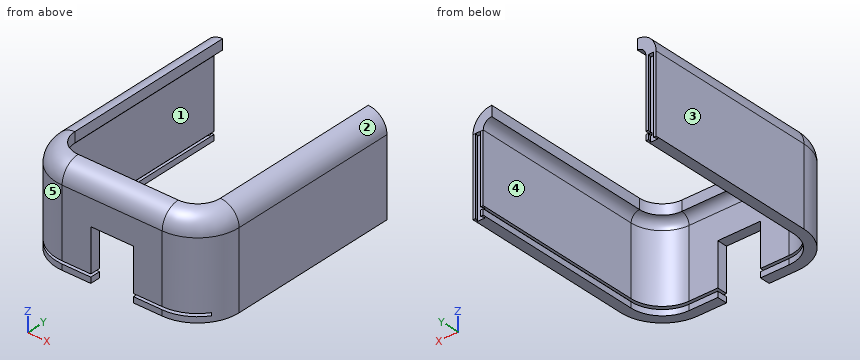
from build123d import *

# Parameters (mm, degrees)
EXTRUDE_1_DEPTH     = 27
CUT_EXTRUDE_1_DEPTH = 1
SKETCH_4_W          = 15
SKETCH_4_H          = 3.6
CUT_EXTRUDE_2_DEPTH = 6
SKETCH_4_2_W        = 15
SKETCH_4_2_H        = 3.6
CUT_EXTRUDE_3_DEPTH = 13


with BuildPart() as part:
    # Sketch 1 → Extrude 1 (new body)
    with BuildSketch(Plane.XY):
        with BuildLine():
            Line((-17.6, -33.659429503), (17.6, -33.659429503))
            ThreePointArc((17.6, -33.659429503), (25.378174593, -30.437604096), (28.6, -22.659429503))
            Line((28.6, -22.659429503), (28.6, 38.340570497))
            Line((28.6, 38.340570497), (29.55, 38.340570497))
            Line((29.55, 38.340570497), (29.040441672, 36.940570497))
            Line((29.040441672, 36.940570497), (31.759558328, 36.940570497))
            Line((31.759558328, 36.940570497), (31.25, 38.340570497))
            Line((31.25, 38.340570497), (32.2, 38.340570497))
            Line((32.2, 38.340570497), (32.2, -22.659429503))
            ThreePointArc((32.2, -22.659429503), (27.923759005, -32.983188509), (17.6, -37.259429503))
            Line((17.6, -37.259429503), (-17.6, -37.259429503))
            ThreePointArc((-17.6, -37.259429503), (-27.923759005, -32.983188509), (-32.2, -22.659429503))
            Line((-32.2, -22.659429503), (-32.2, 38.340570497))
            Line((-32.2, 38.340570497), (-31.25, 38.340570497))
            Line((-31.25, 38.340570497), (-31.759558328, 36.940570497))
            Line((-31.759558328, 36.940570497), (-29.040441672, 36.940570497))
            Line((-29.040441672, 36.940570497), (-29.55, 38.340570497))
            Line((-29.55, 38.340570497), (-28.6, 38.340570497))
            Line((-28.6, 38.340570497), (-28.6, -22.659429503))
            ThreePointArc((-28.6, -22.659429503), (-25.378174593, -30.437604096), (-17.6, -33.659429503))
        make_face()
    extrude(amount=EXTRUDE_1_DEPTH)

    # Sketch 3 → Cut-Extrude 1 (cut)
    with BuildSketch(Plane.XY.offset(3)):
        with BuildLine():
            Line((-28.6, 38.340570497), (-28.6, -22.659429503))
            ThreePointArc((-28.6, -22.659429503), (-25.378174593, -30.437604096), (-17.6, -33.659429503))
            Line((-17.6, -33.659429503), (17.6, -33.659429503))
            ThreePointArc((17.6, -33.659429503), (25.378174593, -30.437604096), (28.6, -22.659429503))
            Line((28.6, -22.659429503), (28.6, 38.340570497))
            Line((28.6, 38.340570497), (29.56, 38.340570497))
            Line((29.56, 38.340570497), (29.56, -22.659429503))
            Line((29.56, -22.659429503), (29.56, -37.259429503))
            Line((29.56, -37.259429503), (-29.56, -37.259429503))
            Line((-29.56, -37.259429503), (-29.56, -22.659429503))
            Line((-29.56, -22.659429503), (-29.56, 38.340570497))
            Line((-29.56, 38.340570497), (-28.6, 38.340570497))
        make_face()
    extrude(amount=-CUT_EXTRUDE_1_DEPTH, mode=Mode.SUBTRACT)

    # Sketch 4 → Cut-Extrude 2 (cut, through all)
    with BuildSketch(Plane.XY.offset(5)):
        with Locations((0, -35.459429503)):
            Rectangle(SKETCH_4_W, SKETCH_4_H)
    extrude(amount=-CUT_EXTRUDE_2_DEPTH, mode=Mode.SUBTRACT)

    # Sweep 4: sweep along a path in Sketch 6
    with BuildLine(Plane.XY.offset(27)) as sweep_4_path:
        Line((-30.4, 38.340570497), (-30.4, 37.968733181))
        Line((-30.4, 37.968733181), (-30.4, -22.659429503))
        ThreePointArc((-30.4, -22.659429503), (-26.650966799, -31.710396303), (-17.6, -35.459429503))
        Line((-17.6, -35.459429503), (17.6, -35.459429503))
        ThreePointArc((17.6, -35.459429503), (26.650966799, -31.710396303), (30.4, -22.659429503))
        Line((30.4, -22.659429503), (30.4, 37.968733181))
        Line((30.4, 37.968733181), (30.4, 38.340570497))
    # Sketch 7 → Sweep 4 (sweep)
    with BuildSketch(Plane(origin=(0, 36.940570497, 0), x_dir=(1, 0, 0), z_dir=(0, 1, 0))):
        with BuildLine():
            Line((-32.2, -27), (-28.6, -27))
            ThreePointArc((-28.6, -27), (-27.721320344, -29.121320344), (-25.6, -30))
            Line((-25.6, -30), (-25.6, -33.6))
            ThreePointArc((-25.6, -33.6), (-30.266904756, -31.666904756), (-32.2, -27))
        make_face()
    sweep(path=sweep_4_path.line)

    # Sketch 4_2 → Cut-Extrude 3 (cut)
    with BuildSketch(Plane.XY.offset(5)):
        with Locations((0, -35.459429503)):
            Rectangle(SKETCH_4_2_W, SKETCH_4_2_H)
    extrude(amount=CUT_EXTRUDE_3_DEPTH, mode=Mode.SUBTRACT)


solid = part.part
Verification items for the finished model (mm, model axes). Face numbers are marked on the shaded views. A direction names the side the tool comes from. Give positions to 0.01 mm unless a question says otherwise; leave off trailing zeros. Write each loop counter-clockwise with the first axis right and the second up, starting at its lowest first coordinate (ties: lowest second). Pieces come first, ordered by that corner, then holes. Notation, with made-up numbers: M 10,69.5 L 42,69.5 A30 cw 42,106.5 Z; hole C 9.25,77 d4. An arc over 180 degrees is marked long. Put each result on its own line as item: value. Start each with the question number.
1. Scan lines: line 1 along X through (y, z) = (-21.5, 24); line 2 along Y through (x, z) = (8, 25); line 3 along Z through (x, y) = (-29, -2). Record each from-to range of solid material in increasing order. Write a range as [from, to].
2. Go/stop test with flat-tipped pins: pin 1 Ø1.5 at (x, z) = (-25, 27.5) entering from +Y; pin 2 Ø12 at (x, z) = (2.5, 13.5) entering from +Y; pin 3 Ø3 at (y, z) = (-35.5, 8) entering from +X; pin 4 Ø10 at (x, z) = (1, 5) entering from +Y. Record where each tip stops, or that it passes through.
3. Draft check along X on the marked faces 1, 2 and 3. Enter one of: +X half, -X half, draft (parallel to the pull), parting line (faces both ways), or undercut.
4. Section check B-B (y = 34). Record the cut outline in (x, z).
5. Section check A-A (x = -12). Record the cut outline in (y, z), and give its area (3 significant figures).
6. Section check C-C (z = 4). Record the cut outline in (x, y).
7. Section check D-D (z = 20.5). Record the cut outline in (x, y), and give its area (3 significant figures).
8. Set-up check for the marked faces 4 and 5: record each of +Z, -Z, +X, -X, +Y, -Y from which the full face is reachable in a straight line by a thin tool's end or side.
Answer list:
1. line 1: [-32.2, -28.6], [28.6, 32.2]
1. line 2: [-37.26, -33.66]
1. line 3: [0, 2], [3, 32.66]
2. pin 1: y = -29.95
2. pin 2: y = -33.66
2. pin 3: x = 26.8
2. pin 4: through
3. face 1: undercut
3. face 2: +X half
3. face 3: -X half
4. outline: M -32.2,0 L -28.6,0 L -28.6,2 L -29.56,2 L -29.56,3 L -28.6,3 L -28.6,27 A3 cw -25.6,30 L -25.6,33.6 A6.6 ccw -32.2,27 Z; M 25.6,30 A3 cw 28.6,27 L 28.6,3 L 29.56,3 L 29.56,2 L 28.6,2 L 28.6,0 L 32.2,0 L 32.2,27 A6.6 ccw 25.6,33.6 Z
5. outline: M -37.26,0 L -33.66,0 L -33.66,2 L -37.26,2 Z; M -37.26,3 L -33.66,3 L -33.66,27 A3 cw -30.66,30 L -30.66,33.6 A6.6 ccw -37.26,27 Z
5. area: 121 mm2
6. outline: M -32.2,-22.66 A14.6 ccw -17.6,-37.26 L -7.5,-37.26 L -7.5,-33.66 L -17.6,-33.66 A11 cw -28.6,-22.66 L -28.6,38.34 L -29.55,38.34 L -29.04,36.94 L -31.76,36.94 L -31.25,38.34 L -32.2,38.34 Z; M 7.5,-37.26 L 17.6,-37.26 A14.6 ccw 32.2,-22.66 L 32.2,38.34 L 31.25,38.34 L 31.76,36.94 L 29.04,36.94 L 29.55,38.34 L 28.6,38.34 L 28.6,-22.66 A11 cw 17.6,-33.66 L 7.5,-33.66 Z
7. outline: M -32.2,-22.66 A14.6 ccw -17.6,-37.26 L 17.6,-37.26 A14.6 ccw 32.2,-22.66 L 32.2,38.34 L 31.25,38.34 L 31.76,36.94 L 29.04,36.94 L 29.55,38.34 L 28.6,38.34 L 28.6,-22.66 A11 cw 17.6,-33.66 L -17.6,-33.66 A11 cw -28.6,-22.66 L -28.6,38.34 L -29.55,38.34 L -29.04,36.94 L -31.76,36.94 L -31.25,38.34 L -32.2,38.34 Z
7. area: 704 mm2
8. face 4: -Z, +Y
8. face 5: +Z, -Z, -X, -Y
